For this review, take the finished solid that the model builds, in its own axes (mm). A direction names the side the tool comes from. Give positions to 0.01 mm unless a question says otherwise; leave off trailing zeros. Write each loop counter-clockwise with the first axis right and the second up, starting at its lowest first coordinate (ties: lowest second). Pieces come first, ordered by that corner, then holes. Notation, with made-up numbers: (55, 56) -> (73, 56) arc R17 ccw to (73, 75) -> close; hole circle Ø2 at (79, 3.25). An arc over 180 degrees is marked (long way). Return JSON: item names as keys, results as strings.
from build123d import *

# Parameters (mm, degrees)
SKETCH1_W               = 8
SKETCH1_H               = 8
BOSS_EXTRUDE1_DEPTH     = 3
CUT_EXTRUDE1_DEPTH      = 12.704699911
CUT_EXTRUDE1_DEPTH_BACK = 12.704699911
CUT_EXTRUDE2_DEPTH      = 11
SKETCH4_R               = 1.75
CUT_EXTRUDE3_DEPTH      = 0.4
SKETCH5_W               = 8
SKETCH5_H               = 1
BOSS_EXTRUDE2_DEPTH     = 2
FILLET1_R               = 4
CUT_EXTRUDE4_DEPTH      = 0.4
CUT_EXTRUDE5_DEPTH      = 0.5


with BuildPart() as part:
    # Sketch1 → Boss-Extrude1 (new body)
    with BuildSketch(Plane(origin=(0, 0, 0), x_dir=(1, 0, 0), z_dir=(0, 1, 0))):
        with Locations((4, 4)):
            Rectangle(SKETCH1_W, SKETCH1_H)
    extrude(amount=BOSS_EXTRUDE1_DEPTH)

    # Sketch2 → Cut-Extrude1 (cut, two sides: drawn at the far end of the back side and taken through both)
    with BuildSketch(Plane.XY.offset(-CUT_EXTRUDE1_DEPTH_BACK)):
        Polygon((0, 0), (0.6, 3), (0, 3), align=None)
        Polygon((8, 0), (7.4, 3), (8, 3), align=None)
    extrude(amount=CUT_EXTRUDE1_DEPTH + CUT_EXTRUDE1_DEPTH_BACK, mode=Mode.SUBTRACT)

    # Sketch3 → Cut-Extrude2 (cut)
    with BuildSketch(Plane(origin=(0, 0, 0), x_dir=(0, 0, -1), z_dir=(1, 0, 0))):
        Polygon((0, 0), (0.6, 3), (0, 3), align=None)
        Polygon((8, 3), (7.4, 3), (8, 0), align=None)
    extrude(amount=CUT_EXTRUDE2_DEPTH, mode=Mode.SUBTRACT)

    # Sketch4 → Cut-Extrude3 (cut)
    with BuildSketch(Plane.XZ):
        with Locations(Location((4, -3.75, 0), (0, 0, 270))):
            Circle(SKETCH4_R)
    extrude(amount=-CUT_EXTRUDE3_DEPTH, mode=Mode.SUBTRACT)

    # Sketch5 → Boss-Extrude2 (add)
    with BuildSketch(Plane.XZ):
        with Locations((4, -7.5)):
            Rectangle(SKETCH5_W, SKETCH5_H)
    extrude(amount=BOSS_EXTRUDE2_DEPTH)

    # Fillet1
    # the kernel refuses this fillet: 4 mm, written as the material it takes off along each edge
    with BuildSketch(Plane(origin=(8, -2, -16.660254038), x_dir=(0, 1, 0), z_dir=(0, 0, 1)), Plane(origin=(0, -2, 1.660254038), x_dir=(0, 1, 0), z_dir=(0, 0, -1))) as fillet1_piece_1:
        with BuildLine():
            CenterArc((4, 3.464101615), FILLET1_R, 180, 60)
            Line((0, 3.464101615), (-0.08, 3.464101615))
            Line((-0.08, 3.464101615), (-0.08, 0))
            Line((-0.08, 0), (0, -0.08))
            ThreePointArc((0, -0.08), (1, -0.08), (1.96, -0.069282032))
            Line((1.96, -0.069282032), (2, 0))
        make_face()
    extrude(amount=18.320508076, mode=Mode.SUBTRACT)

    # Sketch6 → Cut-Extrude4 (cut)
    with BuildSketch(Plane(origin=(0, 3, 0), x_dir=(1, 0, 0), z_dir=(0, 1, 0))):
        Polygon((2.544225106, 2.010567225), (2.544225106, 6.010567225), (5.51858408, 6.010567225), (5.51858408, 5.343900558), (3.313455875, 5.343900558), (3.313455875, 4.472105686), (5.364737926, 4.472105686), (5.364737926, 3.80543902), (3.313455875, 3.80543902), (3.313455875, 2.677233891), (5.569866131, 2.677233891), (5.569866131, 2.010567225), align=None)
    extrude(amount=-CUT_EXTRUDE4_DEPTH, mode=Mode.SUBTRACT)

    # Sketch7 → Cut-Extrude5 (cut)
    with BuildSketch(Plane(origin=(0, 3, 0), x_dir=(1, 0, 0), z_dir=(0, 1, 0))):
        with BuildLine():
            Line((5.822088817, 1.468310464), (6.206704202, 1.515586105))
            add(Edge.make_bspline(
                [(6.206704202, 1.515586105), (6.210025755, 1.491936921), (6.21633053, 1.447047438), (6.235989072, 1.384914698), (6.261652315, 1.330845836), (6.295629161, 1.286544364), (6.334912115, 1.251310519), (6.37872169, 1.226169889), (6.426661607, 1.210315729), (6.460052531, 1.208713548), (6.477136894, 1.207893797)],
                knots=[0, 0, 0, 0, 1.26631894, 2.403651751, 3.447242243, 4.428907923, 5.348362865, 6.231623936, 7.095215805, 8, 8, 8, 8], degree=3))
            add(Edge.make_bspline(
                [(6.477136894, 1.207893797), (6.486366298, 1.208091994), (6.504648304, 1.20848459), (6.531523321, 1.212603697), (6.557345996, 1.219374529), (6.58186155, 1.229117251), (6.605187017, 1.241222715), (6.627629553, 1.255638676), (6.648246393, 1.273643613), (6.668375088, 1.29334292), (6.68623752, 1.315767324), (6.701972196, 1.340096861), (6.715784117, 1.366090219), (6.726489771, 1.394417604), (6.734869896, 1.424465406), (6.740860884, 1.456364057), (6.744506994, 1.489993317), (6.74494315, 1.513039367), (6.74516574, 1.524800849)],
                knots=[0, 0, 0, 0, 0.951760839, 1.885289532, 2.797832748, 3.70117291, 4.60103766, 5.506897018, 6.445598779, 7.420035506, 8.410036365, 9.396193293, 10.407074535, 11.440988179, 12.514285005, 13.622404236, 14.786601276, 16, 16, 16, 16], degree=3))
            add(Edge.make_bspline(
                [(6.74516574, 1.524800849), (6.744331981, 1.546629456), (6.742741494, 1.588269906), (6.730451294, 1.647346431), (6.709137892, 1.699277092), (6.679276772, 1.743130281), (6.643793264, 1.778406879), (6.604044422, 1.8049236), (6.559654571, 1.820157256), (6.528795478, 1.822230353), (6.513194586, 1.823278413)],
                knots=[0, 0, 0, 0, 1.241512862, 2.368321189, 3.414110003, 4.41529485, 5.36642979, 6.245396713, 7.112955941, 8, 8, 8, 8], degree=3))
            add(Edge.make_bspline(
                [(6.513194586, 1.823278413), (6.502087722, 1.822994208), (6.47854234, 1.822391724), (6.441918774, 1.81613185), (6.401980616, 1.80749294), (6.374785766, 1.799182881), (6.360550356, 1.7948329)],
                knots=[0, 0, 0, 0, 0.854525515, 1.811503923, 2.854410343, 4, 4, 4, 4], degree=3))
            Line((6.360550356, 1.7948329), (6.396608048, 2.105329695))
            add(Edge.make_bspline(
                [(6.396608048, 2.105329695), (6.407296254, 2.105146348), (6.428036665, 2.104790564), (6.458323888, 2.107301653), (6.486673662, 2.111886341), (6.513019839, 2.119324972), (6.53738695, 2.128349551), (6.559988104, 2.139688262), (6.580270378, 2.153798702), (6.604965361, 2.175098338), (6.630230561, 2.207014566), (6.6530719, 2.250778884), (6.665798637, 2.300679459), (6.667408863, 2.335629458), (6.668242663, 2.353727131)],
                knots=[0, 0, 0, 0, 0.916749589, 1.778948191, 2.604102396, 3.376994206, 4.124053722, 4.831292757, 5.54010828, 6.238660037, 7.62386988, 9.002523041, 10.447858069, 12, 12, 12, 12], degree=3))
            add(Edge.make_bspline(
                [(6.668242663, 2.353727131), (6.667680515, 2.36913782), (6.666602635, 2.398686702), (6.656933325, 2.440733393), (6.640429824, 2.477855418), (6.617345194, 2.50940841), (6.589028098, 2.535030406), (6.555929861, 2.553963194), (6.518019093, 2.565003531), (6.491366313, 2.566231188), (6.477537535, 2.566868156)],
                knots=[0, 0, 0, 0, 1.146968804, 2.199229744, 3.192297141, 4.153502289, 5.090509175, 6.0173182, 6.971286811, 8, 8, 8, 8], degree=3))
            add(Edge.make_bspline(
                [(6.477537535, 2.566868156), (6.463673911, 2.566182836), (6.436422829, 2.564835732), (6.397428508, 2.551510744), (6.361454157, 2.530893795), (6.329709376, 2.501368407), (6.302195486, 2.464646404), (6.280874208, 2.419861118), (6.265858745, 2.367714197), (6.260698213, 2.33018187), (6.257986253, 2.3104579)],
                knots=[0, 0, 0, 0, 0.889956214, 1.749345552, 2.62404616, 3.543272128, 4.520224035, 5.562553653, 6.719074424, 8, 8, 8, 8], degree=3))
            Line((6.257986253, 2.3104579), (5.873370869, 2.368150208))
            add(Edge.make_bspline(
                [(5.873370869, 2.368150208), (5.879712758, 2.397514751), (5.891852554, 2.453725064), (5.916656, 2.532479948), (5.945759151, 2.602002338), (5.979761878, 2.663071325), (6.020038823, 2.716762155), (6.067859884, 2.763365742), (6.122509575, 2.804234412), (6.183883545, 2.838478774), (6.250614825, 2.865925856), (6.321633047, 2.886240153), (6.396757082, 2.897882068), (6.448117417, 2.899417689), (6.474332407, 2.90020149)],
                knots=[0, 0, 0, 0, 1.220808349, 2.336900656, 3.3513467, 4.279992853, 5.171472476, 6.069835959, 6.985198729, 7.938095762, 8.919113729, 9.91246339, 10.934493858, 12, 12, 12, 12], degree=3))
            add(Edge.make_bspline(
                [(6.474332407, 2.90020149), (6.496795991, 2.899690329), (6.540685792, 2.898691614), (6.604687523, 2.890097866), (6.665244055, 2.876137228), (6.722439804, 2.856388937), (6.776539911, 2.831244798), (6.826641223, 2.799609265), (6.873794781, 2.763093379), (6.901724377, 2.73467508), (6.915838817, 2.720313669)],
                knots=[0, 0, 0, 0, 1.096978699, 2.143298912, 3.148181587, 4.128190255, 5.094201205, 6.055441919, 7.017302331, 8, 8, 8, 8], degree=3))
            add(Edge.make_bspline(
                [(6.915838817, 2.720313669), (6.926741328, 2.708075606), (6.948274918, 2.683904162), (6.976233385, 2.645150995), (6.999633117, 2.604882958), (7.019482141, 2.563940258), (7.034243104, 2.52137348), (7.04524752, 2.477850813), (7.051783755, 2.43298662), (7.05249893, 2.402626167), (7.052858048, 2.387380977)],
                knots=[0, 0, 0, 0, 1.065582675, 2.104636323, 3.101288825, 4.092056841, 5.059084899, 6.026073946, 7.008813224, 8, 8, 8, 8], degree=3))
            add(Edge.make_bspline(
                [(7.052858048, 2.387380977), (7.052074688, 2.365937591), (7.050530541, 2.323668734), (7.036361111, 2.262180096), (7.013586987, 2.204054017), (6.982096895, 2.149068456), (6.941041129, 2.097733658), (6.890499978, 2.050511525), (6.831958555, 2.005600039), (6.787958464, 1.980231405), (6.765197792, 1.967108541)],
                knots=[0, 0, 0, 0, 0.957571776, 1.887550067, 2.804499428, 3.740591036, 4.709432777, 5.731457079, 6.826512349, 8, 8, 8, 8], degree=3))
            add(Edge.make_bspline(
                [(6.765197792, 1.967108541), (6.778741549, 1.963844189), (6.805468134, 1.957402478), (6.844077906, 1.94426987), (6.880236126, 1.927424278), (6.914828375, 1.908914943), (6.946996208, 1.886966635), (6.977363151, 1.862646466), (7.00476785, 1.834549826), (7.03102769, 1.804865641), (7.053982146, 1.772288453), (7.074722978, 1.738388398), (7.091382436, 1.702338355), (7.105631297, 1.665065232), (7.116248441, 1.625966572), (7.124562393, 1.585334894), (7.128729622, 1.542917296), (7.129427921, 1.514124194), (7.129781125, 1.499560464)],
                knots=[0, 0, 0, 0, 1.037381978, 2.047118658, 3.030848314, 4.005687143, 4.965748246, 5.927353932, 6.897971669, 7.885165084, 8.876109723, 9.862099733, 10.840989857, 11.829385213, 12.830906716, 13.855042526, 14.915067134, 16, 16, 16, 16], degree=3))
            add(Edge.make_bspline(
                [(7.129781125, 1.499560464), (7.129332308, 1.478289376), (7.12844718, 1.43633993), (7.11872513, 1.374773186), (7.10395436, 1.3156035), (7.083598929, 1.25859183), (7.056376257, 1.204435717), (7.023823759, 1.152375398), (6.985054773, 1.102929453), (6.940845684, 1.056472589), (6.892539484, 1.013951446), (6.84063463, 0.97660242), (6.785900139, 0.944991177), (6.728022396, 0.9191431), (6.667504686, 0.899031537), (6.603826037, 0.885208987), (6.537502989, 0.875987213), (6.49212598, 0.875040406), (6.469124074, 0.874560464)],
                knots=[0, 0, 0, 0, 1.006520189, 1.984993146, 2.943645202, 3.891894145, 4.845023195, 5.808336607, 6.795092628, 7.815033679, 8.841288157, 9.838185905, 10.83832808, 11.829129029, 12.835072876, 13.85234392, 14.911338897, 16, 16, 16, 16], degree=3))
            add(Edge.make_bspline(
                [(6.469124074, 0.874560464), (6.447326457, 0.874925903), (6.404510806, 0.875643711), (6.341832261, 0.884147308), (6.281800208, 0.896657101), (6.224765045, 0.914957582), (6.170229951, 0.937498647), (6.119224255, 0.966556317), (6.070434994, 0.999582769), (6.02545616, 1.03827062), (5.983635573, 1.080436419), (5.946901196, 1.126807021), (5.914165969, 1.175902437), (5.886010541, 1.228157933), (5.862670856, 1.283709297), (5.844497682, 1.342413141), (5.830004226, 1.404089696), (5.824763645, 1.446608551), (5.822088817, 1.468310464)],
                knots=[0, 0, 0, 0, 1.077528213, 2.11651914, 3.123276654, 4.10732375, 5.075386463, 6.036572488, 7.005896639, 7.98540975, 8.966414275, 9.939311093, 10.906719916, 11.882103104, 12.870994428, 13.882228509, 14.919075059, 16, 16, 16, 16], degree=3))
        make_face()
    extrude(amount=-CUT_EXTRUDE5_DEPTH, mode=Mode.SUBTRACT)


solid = part.part
1. Add section C-C, the plane z = -5. State the section outline as (x, y) points, plus the area to 3 significant figures.
Results found:
{"outline": "(0, 0) -> (2.78, 0) -> (2.78, 0.4) -> (5.22, 0.4) -> (5.22, 0) -> (8, 0) -> (7.4, 3) -> (3.31, 3) -> (3.31, 2.6) -> (2.54, 2.6) -> (2.54, 3) -> (0.6, 3) -> close", "area": "20.9 mm²"}
2. For pin 1 (3 mm diameter, centred on x = 4, z = -3.75, fed in from -Y); pin 2 (1 mm diameter, centred on y = 2.5, z = -1.5, fed in from +X); pin 3 (1.6 mm diameter, centred on x = 5, y = -1, fed in from +Z), all flat-tipped, find the tip position at first contact; note any pin that passes through.
Results found:
{"pin 1": "stops at y = 0.4", "pin 2": "stops at x = 7.6", "pin 3": "stops at z = -7"}
3. The part is to be moulded in two halves that separate along Z. For faces 4 (the flat face through (3.9, 1.5, -0.3)), 5 (the flat face through (0.3, 1.5, -4.1)), 6 (the flat face through (4, 0.4, -4)), say which applies: +Z half, -Z half, draft (parallel to the pull), parting line (faces both ways), or undercut.
Results found:
{"face 4": "+Z half", "face 5": "draft", "face 6": "undercut"}
4. Add section B-B, the plane y = 0.65. State the section outline as (x, z) points, plus the area to 3 significant figures.
Results found:
{"outline": "(0.13, -7.87) -> (7.87, -7.87) -> (7.87, -0.13) -> (0.13, -0.13) -> close", "area": "59.9 mm²"}
5. To check wall thickness, follow probe 1 along Y at (x, z) = (4.75, -3); probe 2 along Y at (x, z) = (4, -4.25); probe 3 along X at (y, z) = (2.75, -5.75). State the ranges of each line that lie inside material, in increasing order.
Results found:
{"probe 1": "y = 0.4 to 3", "probe 2": "y = 0.4 to 2.6", "probe 3": "x = 0.55 to 2.54, 5.52 to 7.45"}
6. Add section D-D, the plane x = 5. State the section outline as (y, z) points.
Results found:
{"outline": "(-1.97, -8) -> (0, -8) -> (3, -7.4) -> (3, -6.01) -> (2.6, -6.01) -> (2.6, -5.34) -> (3, -5.34) -> (3, -4.47) -> (2.6, -4.47) -> (2.6, -3.81) -> (3, -3.81) -> (3, -2.68) -> (2.6, -2.68) -> (2.6, -2.01) -> (3, -2.01) -> (3, -0.6) -> (0, 0) -> (0, -2.31) -> (0.4, -2.31) -> (0.4, -5.19) -> (0, -5.19) -> (0, -7) -> (-1.97, -7) -> close"}
7. For faces 1 (the flat face through (3, 0, -2)), 2 (the flat face through (3.9, 1.5, -7.7)), 3 (the cylindrical face through (2.94, 0.2, -2.36)), list the 3-axis set-ups (+Z, -Z, +X, -X, +Y, -Y) from which the entire face can be reached by the end or side of a thin tool; tool diameter is ignored.
Results found:
{"face 1": "+Z, +X, -X, -Y", "face 2": "-Z, +X, -X, +Y", "face 3": "-Y"}
8. Add section A-A, the plane x = 4. State the section outline as (y, z) points.
Results found:
{"outline": "(-2, -8) -> (0, -8) -> (3, -7.4) -> (3, -6.01) -> (2.6, -6.01) -> (2.6, -5.34) -> (3, -5.34) -> (3, -4.47) -> (2.6, -4.47) -> (2.6, -3.81) -> (3, -3.81) -> (3, -2.68) -> (2.6, -2.68) -> (2.6, -2.01) -> (3, -2.01) -> (3, -0.6) -> (0, 0) -> (0, -2) -> (0.4, -2) -> (0.4, -5.5) -> (0, -5.5) -> (0, -7) -> (-2, -7) -> close"}
